Could you check a few things on this model? Use its own coordinates, in mm. A direction names the side the tool comes from. Coordinates: 2 decimals unless noted, no trailing zeros. Write each loop counter-clockwise with the first axis right and the second up, starting at its lowest first coordinate (ties: lowest second). Pieces come first, ordered by that corner, then holes.
Item 1: I want a section at D-D on x = -32.5. Please give me the cut outline in (y, z), then the cut area to 3 significant figures.
Item 2: Thinking about a two-plate mould opening in Z: for faces 3 (the flat face through (21, -21, -26)), 4 (the cylindrical face through (95.38, 30.04, 27.97)), 5 (the flat face through (21, -21, 26)), which applies, +Z half, -Z half, draft (parallel to the pull), parting line (faces both ways), or undercut?
Item 3: For P1, Ø19, axis at x = 0, y = 0, coming from the -Z side; P2, Ø1.5, axis at y = -15, z = -13, coming from the +X side; P3, Ø5, axis at x = 15.5, z = -17, coming from the +Y side, each with a flat end and sliding along its axis, tell me the tip position at first contact or that it passes through.
Item 4: I want a section at A-A on x = 0. Please give me the cut outline in (y, z).
Item 5: If I drill on probe 1 along Z at (x, y) = (64, 37.5); probe 2 along Y at (x, z) = (0, 18); probe 3 along Y at (x, z) = (20, 17), over which ranges is the centre line in solid material (lowest first)?
Item 6: Which directions (+Z, -Z, +X, -X, +Y, -Y) give clear straight access to the entire face, cutting with the end or side of a thin tool? Please do faces 1 (the cylindrical face through (-5.961, -26.846, -0.364)), 2 (the cylindrical face through (95.38, 30.04, -27.97)).
Item 7: I want a section at C-C on z = -15.5. Please give me the cut outline in (x, y).
from build123d import *

# Parameters (mm, degrees)
SKETCH1_R           = 100
SKETCH1_R_2         = 26.25
SKETCH1_R_3         = 16.000000004
BOSS_EXTRUDE1_DEPTH = 30
SKETCH2_R           = 100
SKETCH2_R_2         = 27.5
CUT_EXTRUDE1_DEPTH  = 26


with BuildPart() as part:
    # Sketch1 → Boss-Extrude1 (new, symmetric)
    # profile 1 of 2: a face of its own
    with BuildSketch(Plane.XY):
        Circle(SKETCH1_R)
        Circle(SKETCH1_R_2, mode=Mode.SUBTRACT)
    # profile 2 of 2: a face of its own
    with BuildSketch(Plane.XY):
        Circle(SKETCH1_R_2)
        Circle(SKETCH1_R_3, mode=Mode.SUBTRACT)
    extrude(amount=BOSS_EXTRUDE1_DEPTH, both=True)

    # Sketch2 → Cut-Extrude1 (cut, symmetric)
    with BuildSketch(Plane.XY):
        Circle(SKETCH2_R)
        Circle(SKETCH2_R_2, mode=Mode.SUBTRACT)
    extrude(amount=CUT_EXTRUDE1_DEPTH, both=True, mode=Mode.SUBTRACT)


solid = part.part
Response values:
1. outline: (-94.57, -30) - (94.57, -30) - (94.57, -26) - (-94.57, -26) - close; (-94.57, 26) - (94.57, 26) - (94.57, 30) - (-94.57, 30) - close
1. area: 1,510 mm2
2. face 3: undercut
2. face 4: draft
2. face 5: undercut
3. P1: passes through
3. P2: stops at x = 23.52
3. P3: stops at y = 24.23
4. outline: (-100, -30) - (-16, -30) - (-16, 30) - (-100, 30) - (-100, 26) - (-27.5, 26) - (-27.5, -26) - (-100, -26) - close; (16, -30) - (100, -30) - (100, -26) - (27.5, -26) - (27.5, 26) - (100, 26) - (100, 30) - (16, 30) - close
5. probe 1: z = -30 to -26, 26 to 30
5. probe 2: y = -27.5 to -16, 16 to 27.5
5. probe 3: y = -18.87 to 18.87
6. face 1: none
6. face 2: +Z, -Z
7. outline: circle Ø55 at (0, 0); hole circle Ø32 at (0, 0)
